Can you work these out from the model? Positions are in its coordinate system, mm. Face numbers are marked on the shaded views. Coordinates: 2 decimals unless noted, no trailing zeros. Loops run counter-clockwise (first coordinate to the right, second up) from the corner with the lowest first, then second, coordinate; pieces in that order, holes last. Notation, with made-up numbers: M 44,-8.5 L 59,-8.5 A16 cw 59,0.5 Z; hole C -19,25.5 d7. An arc over 180 degrees is marked long. Answer as a JSON object with one key per item and string values. Group by question number.
Item 1: Suppose I cut it at B-B (z = 5). Write out the boundary of the cut face in (x, y), then the cut area to 3 significant figures.
Item 2: I'm going to push a flat-ended pin straight in: pin 1 Ø12 at (x, z) = (-61.5, 9) entering from +Y. Where does the tip first touch, or does it pass through?
Item 3: Suppose I cut it at A-A (x = 1.5). Write out the boundary of the cut face in (y, z).
Item 4: If I drill on line 1 (Y direction, x = -30.5, z = 35.5); line 2 (Y direction, x = -37, z = 9); line 3 (X direction, y = 0.5, z = 46), over which ranges is the centre line in solid material (lowest first)?
Item 5: We'd pull the mould along Z, two halves only. Please class the marked faces 1, 2, 3 and 4: +Z half, -Z half, draft (parallel to the pull), parting line (faces both ways), or undercut.
Item 6: Suppose I cut it at D-D (x = -45). Write out the boundary of the cut face in (y, z), then the cut area to 3 significant figures.
Item 7: Suppose I cut it at C-C (x = -27.5). Write out the boundary of the cut face in (y, z).
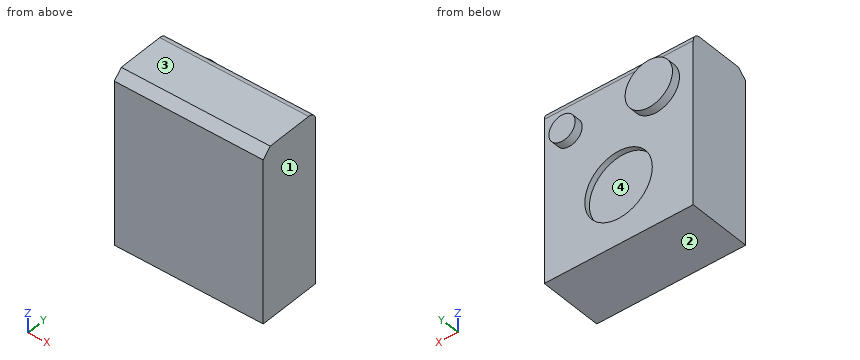
```python
from build123d import *

# Parameters (mm, degrees)
F0_W     = 89.529717
F0_H     = 103.844382
F1_DEPTH = 38.1
F2_SIZE  = 5.08
F3_R     = 5.08
F4_R     = 20.287785
F5_DEPTH = 3.302
F6_R     = 7.910996
F6_R_2   = 14.245045
F7_DEPTH = 5.08


with BuildPart() as f1:
    # F0 (on Front) → F1 (new body)
    with BuildSketch(Plane.XZ):
        with Locations((-32.89539, 12.548234)):
            Rectangle(F0_W, F0_H)
    extrude(amount=F1_DEPTH)

    # F2
    f2_edges = [f1.edges().sort_by_distance(p)[0] for p in [
        (-32.895389, -38.1, 64.470425),
    ]]
    chamfer(f2_edges, length=F2_SIZE)

    # F3
    f3_edges = [f1.edges().sort_by_distance(p)[0] for p in [
        (-32.895389, 0, 64.470425),
    ]]
    fillet(f3_edges, radius=F3_R)

    # F4 (on face) → F5 (cut)
    with BuildSketch(Plane(origin=(0, 0, 0), x_dir=(-1, 0, 0), z_dir=(0, 1, 0))):
        with Locations((32.772042, -3.602346)):
            Circle(F4_R)
    extrude(amount=-F5_DEPTH, mode=Mode.SUBTRACT)

    # F6 (on face) → F7 (join)
    with BuildSketch(Plane(origin=(0, 0, 0), x_dir=(-1, 0, 0), z_dir=(0, 1, 0))):
        with Locations((3.005289, 43.038554)):
            Circle(F6_R)
        with Locations((55.144507, 42.090569)):
            Circle(F6_R_2)
    extrude(amount=F7_DEPTH)


solid = f1.part
```
From the geometry:
{
 "1": {"outline": "M -77.66,-38.1 L 11.87,-38.1 L 11.87,0 L -14.4,0 L -14.4,-3.3 L -51.15,-3.3 L -51.15,0 L -77.66,0 Z", "area": "3,290 mm2"},
 "2": {"pin 1": "y = 0"},
 "3": {"outline": "M -38.1,-39.37 L 0,-39.37 L 0,36.54 L 5.08,36.54 L 5.08,49.54 L 0,49.54 L 0,59.39 A5.08 ccw -5.08,64.47 L -33.02,64.47 L -38.1,59.39 Z"},
 "4": {"line 1": "-38.1 to 0", "line 2": "-38.1 to -3.3", "line 3": "-68.84 to -41.45, -10.34 to 4.33"},
 "5": {"face 1": "draft", "face 2": "-Z half", "face 3": "+Z half", "face 4": "undercut"},
 "6": {"outline": "M -38.1,-39.37 L 0,-39.37 L 0,-19.79 L -3.3,-19.79 L -3.3,12.59 L 0,12.59 L 0,32.09 L 5.08,32.09 L 5.08,52.09 L 0,52.09 L 0,59.39 A5.08 ccw -5.08,64.47 L -33.02,64.47 L -38.1,59.39 Z", "area": "3,930 mm2"},
 "7": {"outline": "M -38.1,-39.37 L 0,-39.37 L 0,-23.19 L -3.3,-23.19 L -3.3,15.99 L 0,15.99 L 0,59.39 A5.08 ccw -5.08,64.47 L -33.02,64.47 L -38.1,59.39 Z"}
}
